from build123d import *

# Parameters (mm, degrees)
F0_W     = 25.4
F0_H     = 101.6
F0_R     = 3.175
F1_DEPTH = 25.4


with BuildPart() as f1:
    # F0 (on Front) → F1 (new body)
    with BuildSketch(Plane.XZ):
        with Locations((-88.9, 50.8)):
            Rectangle(F0_W, F0_H)
        with Locations((-88.9, 12.7)):
            Circle(F0_R, mode=Mode.SUBTRACT)
        Polygon((-76.2, 0), (-50.8, 0), (-50.8, 127), (-76.2, 127), (-76.2, 101.6), align=None)
        Polygon((-50.8, 0), (-25.4, 0), (-25.4, 152.4), (-50.8, 152.4), (-50.8, 127), align=None)
        Polygon((-25.4, 0), (0, 0), (0, 177.8), (-25.4, 177.8), (-25.4, 152.4), align=None)
        Polygon((0, 177.8), (0, 0), (25.4, 0), (25.4, 152.4), (25.4, 177.8), align=None)
        Polygon((25.4, 152.4), (25.4, 0), (50.8, 0), (50.8, 127), (50.8, 152.4), align=None)
        Polygon((50.8, 127), (50.8, 0), (76.2, 0), (76.2, 101.6), (76.2, 127), align=None)
        with Locations((88.9, 50.8)):
            Rectangle(F0_W, F0_H)
        with Locations((88.9, 12.7)):
            Circle(F0_R, mode=Mode.SUBTRACT)
    extrude(amount=F1_DEPTH)


solid = f1.part
The listing builds one solid part. Answer for the finished solid, in the listing's coordinates (mm). A direction names the side the tool comes from. Round coordinates to 2 decimals unless told otherwise and drop trailing zeros. Write each loop counter-clockwise with the first axis right and the second up, starting at its lowest first coordinate (ties: lowest second). Pieces come first, ordered by that corner, then holes. Notation, with made-up numbers: M 30.25,25.25 L 84.25,25.25 A10 ccw 84.25,37.25 Z; hole C 39.5,12 d4. An arc over 180 degrees is marked long. Write each question's results on one line, items separated by ' | '. Start each with the question number.
(1) The part is cut by section C-C, the plane y = -9.75. Write down the section's boundary in (x, z) (3 decimals).
(2) The part is cut by section B-B, the plane x = -88.9. Write down the section's boundary in (y, z) (3 decimals), and give its area (3 significant figures).
(3) For faces 4 (the flat face through (-89, -13, 101.6)), 5 (the flat face through (-1, -13, 0)), 6 (the flat face through (89, -13, 101.6)), determine the directions among +Z, -Z, +X, -X, +Y, -Y from which every point of the face is accessible in a straight line to the end or side of a thin tool.
(4) Determine the mould class of faces 1 (the cylindrical face through (-92.07, -12.52, 12.84)), 2 (the flat face through (64, -13, 127)), 3 (the flat face through (-76.2, -13, 114)) for opening direction Z: +Z half, -Z half, draft (parallel to the pull), parting line (faces both ways), or undercut.
(5) The part is cut by section D-D, the plane z = 133. Write down the section's boundary in (x, y), and give its area (3 significant figures).
(6) The part is cut by section A-A, the plane z = 12.7. Write down the section's boundary in (x, y) (3 decimals), and give its area (3 significant figures).
(7) Find the intervals of material crossed by line 1 (Z direction, x = -88.9, y = -17) (3 decimals); line 2 (X direction, y = -16.5, z = 161); line 3 (X direction, y = -15, z = 126), in increasing order.
(8) Each of these flat-tipped pins is pushed along its axis until it touches: P1, Ø7.5, axis at y = -17, z = 160.5, coming from the +X side; P2, Ø12.5, axis at y = -15, z = 108.5, coming from the -X side; P3, Ø7.5, axis at x = -85, y = -8, coming from the +Z side. Where does it stop, or does it pass through?
Worked answers:
1) outline: M -101.6,0 L 101.6,0 L 101.6,101.6 L 76.2,101.6 L 76.2,127 L 50.8,127 L 50.8,152.4 L 25.4,152.4 L 25.4,177.8 L -25.4,177.8 L -25.4,152.4 L -50.8,152.4 L -50.8,127 L -76.2,127 L -76.2,101.6 L -101.6,101.6 Z; hole C -88.9,12.7 d6.35; hole C 88.9,12.7 d6.35
2) outline: M -25.4,0 L 0,0 L 0,9.525 L -25.4,9.525 Z; M -25.4,15.875 L 0,15.875 L 0,101.6 L -25.4,101.6 Z | area: 2,420 mm²
3) face 4: +Z, -X, +Y, -Y | face 5: -Z, +X, -X, +Y, -Y | face 6: +Z, +X, +Y, -Y
4) face 1: undercut | face 2: +Z half | face 3: draft
5) outline: M -50.8,-25.4 L 50.8,-25.4 L 50.8,0 L -50.8,0 Z | area: 2,580 mm²
6) outline: M -101.6,-25.4 L -92.075,-25.4 L -92.075,0 L -101.6,0 Z; M -85.725,-25.4 L 85.725,-25.4 L 85.725,0 L -85.725,0 Z; M 92.075,-25.4 L 101.6,-25.4 L 101.6,0 L 92.075,0 Z | area: 4,840 mm²
7) line 1: z = 0 to 9.525, 15.875 to 101.6 | line 2: x = -25.4 to 25.4 | line 3: x = -76.2 to 76.2
8) P1: stops at x = 25.4 | P2: stops at x = -76.2 | P3: stops at z = 101.6
